from build123d import *

# Parameters (mm, degrees)
F1_DEPTH = 4
F2_T     = -1.5
F5_DEPTH = 1
F6_R     = 3
F7_R     = 1.5
F9_DEPTH = 25


with BuildPart() as f1:
    # F0 (on Top) → F1 (new body)
    with BuildSketch(Plane.XY):
        with BuildLine():
            ThreePointArc((-6.5, 0), (-1.9038059223, 1.9038059223), (0, 6.5))
            Line((0, 6.5), (0, 47.4878030638))
            ThreePointArc((0, 47.4878030638), (-35.8449314192, 35.8449314192), (-47.4878030638, 0))
            Line((-47.4878030638, 0), (-13, 0))
            Line((-13, 0), (-6.5, 0))
        make_face()
    extrude(amount=F1_DEPTH)

    # F2
    f2_openings = [f1.faces().sort_by_distance(p)[0] for p in [
        (-21.274509, 21.274509, 4),
        (-21.274509, 21.274509, 0),
    ]]
    offset(amount=F2_T, openings=f2_openings)

    # F4 (on offset) → F5 (join)
    with BuildSketch(Plane.XY.offset(1.5)):
        with BuildLine():
            Line((-46.186269666, 1.5), (-6.5, 1.5))
            ThreePointArc((-6.5, 1.5), (-2.9644660941, 2.9644660941), (-1.5, 6.5))
            Line((-1.5, 6.5), (-1.5, 46.186269666))
            ThreePointArc((-1.5, 46.186269666), (-34.7842712475, 34.7842712475), (-46.186269666, 1.5))
        make_face()
    extrude(amount=F5_DEPTH)

    # F6
    f6_edges = [f1.edges().sort_by_distance(p)[0] for p in [
        (0, 47.487803, 2),
        (-47.487803, 0, 2),
    ]]
    fillet(f6_edges, radius=F6_R)

    # F7
    f7_edges = [f1.edges().sort_by_distance(p)[0] for p in [
        (-1.5, 46.18627, 0.75),
        (-46.18627, 1.5, 0.75),
        (-46.18627, 1.5, 3.25),
        (-1.5, 46.18627, 3.25),
    ]]
    fillet(f7_edges, radius=F7_R)

    # F8 (on face) → F9 (cut)
    with BuildSketch(Plane.XY.offset(4)):
        with BuildLine():
            ThreePointArc((-6.5, 1.5), (-2.9644660941, 2.9644660941), (-1.5, 6.5))
            ThreePointArc((-1.5, 6.5), (-10.0355339059, 10.0355339059), (-6.5, 1.5))
        make_face()
    extrude(amount=-F9_DEPTH, mode=Mode.SUBTRACT)


solid = f1.part
For this review, take the finished solid that the model builds, in its own axes (mm). A direction names the side the tool comes from. Round coordinates to 2 decimals unless told otherwise and drop trailing zeros. Loops run counter-clockwise (first coordinate to the right, second up) from the corner with the lowest first, then second, coordinate; pieces in that order, holes last. Notation, with made-up numbers: (27, 22) - (41, 22) arc R10 cw to (41, 29) - close; hole circle Ø3 at (-10.5, 82.25). An arc over 180 degrees is marked (long way). Use one line per item in the form item = value.
Item 1: Consider section A-A on z = 3.05. Write out the cut boundary in (x, y).
Answers:
outline = (-47.83, 2.73) arc R3 ccw to (-44.84, 0) - (-6.5, 0) arc R6.5 ccw to (0, 6.5) - (0, 44.84) arc R3 ccw to (-2.73, 47.83) arc R41.5 ccw to start; hole (-46.33, 2.86) arc R1.5 ccw to (-44.84, 1.5) - (-6.5, 1.5) arc R5 ccw to (-1.5, 6.5) - (-1.5, 44.84) arc R1.5 ccw to (-2.86, 46.33) arc R40 ccw to start
Item 2: Consider section D-D on x = -30. Write out the cut boundary in (y, z).
Answers:
outline = (0, 0) - (1.5, 0) - (1.5, 1.5) - (38.87, 1.5) - (38.87, 0) - (40.71, 0) - (40.71, 4) - (38.87, 4) - (38.87, 2.5) - (1.5, 2.5) - (1.5, 4) - (0, 4) - close
Item 3: Consider section C-C on y = 35.5. Write out the cut boundary in (x, z), then the cut area to 3 significant figures.
Answers:
outline = (-36.19, 0) - (-34.05, 0) - (-34.05, 1.5) - (-1.5, 1.5) - (-1.5, 0) - (0, 0) - (0, 4) - (-1.5, 4) - (-1.5, 2.5) - (-34.05, 2.5) - (-34.05, 4) - (-36.19, 4) - close
area = 47.1 mm^2
Item 4: Clearance check with flat-ended pins moving along their axes: P1, Ø1.6, axis at x = -26.5, z = 3.5, coming from the +Y side; P2, Ø1.2, axis at y = 34, z = 0.5, coming from the -X side; P3, Ø13.5, axis at x = -15, y = 26, coming from the +Z side; P4, Ø9, axis at x = -6.5, y = 6.5, coming from the -Z side. State where each tip first meets the part, or that it passes through.
Answers:
P1 = 43.29
P2 = -38.1
P3 = 2.5
P4 = through
Item 5: Mouldability with a two-part tool opening along Y and no side actions: class faces 1 (the flat face through (-1.5, 25, 1)), 2 (the cylindrical face through (-0.764, 46.84, 2.028)), 3 (the flat face through (0, 25, 2)) as +Y half, -Y half, draft (parallel to the pull), parting line (faces both ways), or undercut.
Answers:
face_1 = undercut
face_2 = +Y half
face_3 = draft
Item 6: Consider section B-B on x = -9.5. Write out the cut boundary in (y, z), then the cut area to 3 significant figures.
Answers:
outline = (0, 0) - (1.5, 0) - (1.5, 1.5) - (2.5, 1.5) - (2.5, 2.5) - (1.5, 2.5) - (1.5, 4) - (0, 4) - close; (10.5, 1.5) - (46.39, 1.5) - (46.39, 0) - (47.89, 0) - (47.89, 4) - (46.39, 4) - (46.39, 2.5) - (10.5, 2.5) - close
area = 48.9 mm^2
Item 7: For line 1 (X direction, y = 6.5, z = 2.7); line 2 (Y direction, x = -6.5, z = 1.4); line 3 (X direction, y = 6.5, z = 1.85), list the stretches that pass through material, from the lowest coordinate up.
Answers:
line_1 = -48 to -46.5, -1.5 to 0
line_2 = 0 to 1.5, 46.5 to 48
line_3 = -48 to -11.5, -1.5 to 0
Item 8: Tool access review of faces 4 (the flat face through (-26, 1.5, 3)), 5 (the flat face through (-26, 0, 2)), 6 (the flat face through (-24, 24, 1.5)): name each direction out of +Z, -Z, +X, -X, +Y, -Y from which nothing blocks a thin tool from reaching the whole face with its end or side.
Answers:
face_4 = +Z
face_5 = +Z, -Z, +X, -X, -Y
face_6 = -Z
